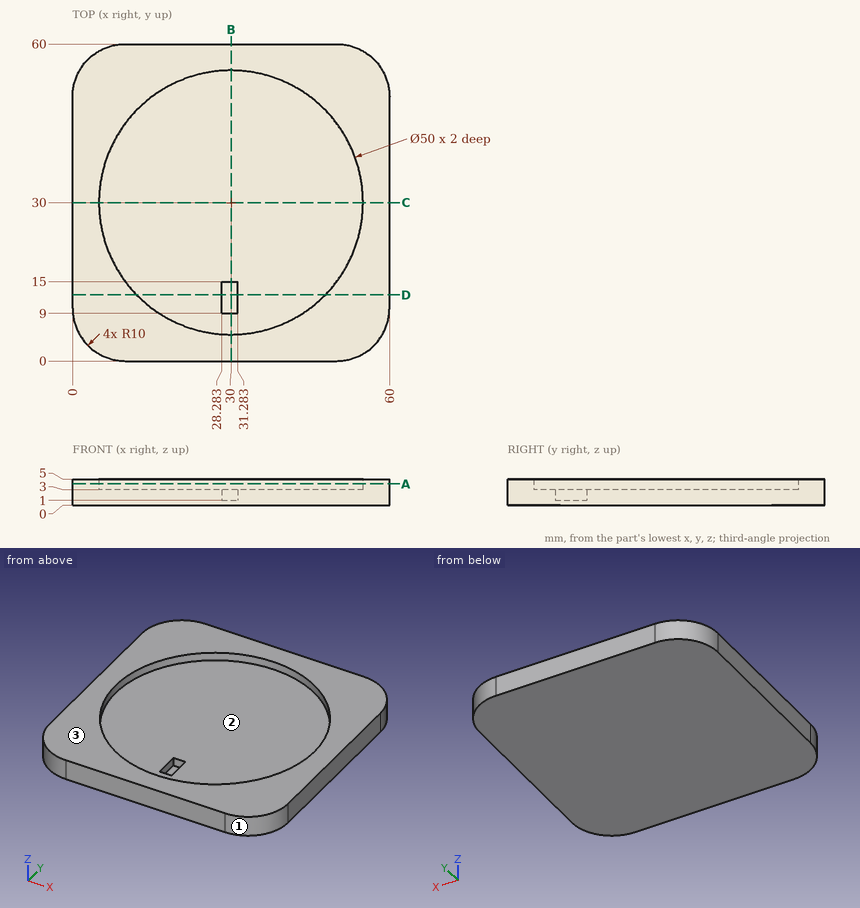
Check sheet for the drawn part. Datum: minimum x, y, z corner. Units: mm. Give positions to 0.01 mm unless a question says otherwise; leave off trailing zeros. Order: outer loops, then holes, each group sorted by start corner. A loop starts at its lowest first (then second) coordinate and runs counter-clockwise, first axis right, second up. Notation, with made-up numbers: (16.5, -19.5) - (23.5, -19.5) arc R26 ccw to (23.5, 13.5) - close; hole circle Ø8 at (37, 55.25). An arc over 180 degrees is marked (long way). Write item = value, one per line. Start each with the question number.
1) Section check D-D (y = 12.5). Enter the section's corners in (x, z).
2) Gauge pin test, flat end, axial feed: pin 1 Ø2.5 at (x, y) = (29.5, 11.5) entering from +Z. Record the tip position at first contact, or that the pin passes through.
3) Section check B-B (x = 30). Enter the section's corners in (y, z).
4) Scan lines: L1, parallel to Y at x = 30, z = 4.35; L2, parallel to Z at x = 22.5, y = 25.5; L3, parallel to Y at x = 40.5, z = 4.45. Record each from-to range of solid material in increasing order.
5) Draft check along Y on the marked faces 1, 2 and 3. Enter one of: released by +Y, released by -Y, zero draft, split by the parting line, or undercut.
6) Section check C-C (y = 30). Enter the section's corners in (x, z), then the cut area to 3 significant figures.
7) Section check A-A (z = 4.1). Enter the section's corners in (x, y), then the cut area to 3 significant figures.
Geometry check:
q1.outline = (0, 0) - (60, 0) - (60, 5) - (47.85, 5) - (47.85, 3) - (31.28, 3) - (31.28, 1) - (28.28, 1) - (28.28, 3) - (12.15, 3) - (12.15, 5) - (0, 5) - close
q2.pin_1 = 3
q3.outline = (0, 0) - (60, 0) - (60, 5) - (55, 5) - (55, 3) - (15, 3) - (15, 1) - (9, 1) - (9, 3) - (5, 3) - (5, 5) - (0, 5) - close
q4.L1 = 0 to 5, 55 to 60
q4.L2 = 0 to 3
q4.L3 = 0 to 7.31, 52.69 to 60
q5.face_1 = released by -Y
q5.face_2 = undercut
q5.face_3 = zero draft
q6.outline = (0, 0) - (60, 0) - (60, 5) - (55, 5) - (55, 3) - (5, 3) - (5, 5) - (0, 5) - close
q6.area = 200 mm2
q7.outline = (0, 10) arc R10 ccw to (10, 0) - (50, 0) arc R10 ccw to (60, 10) - (60, 50) arc R10 ccw to (50, 60) - (10, 60) arc R10 ccw to (0, 50) - close; hole circle Ø50 at (30, 30)
q7.area = 1,550 mm2
